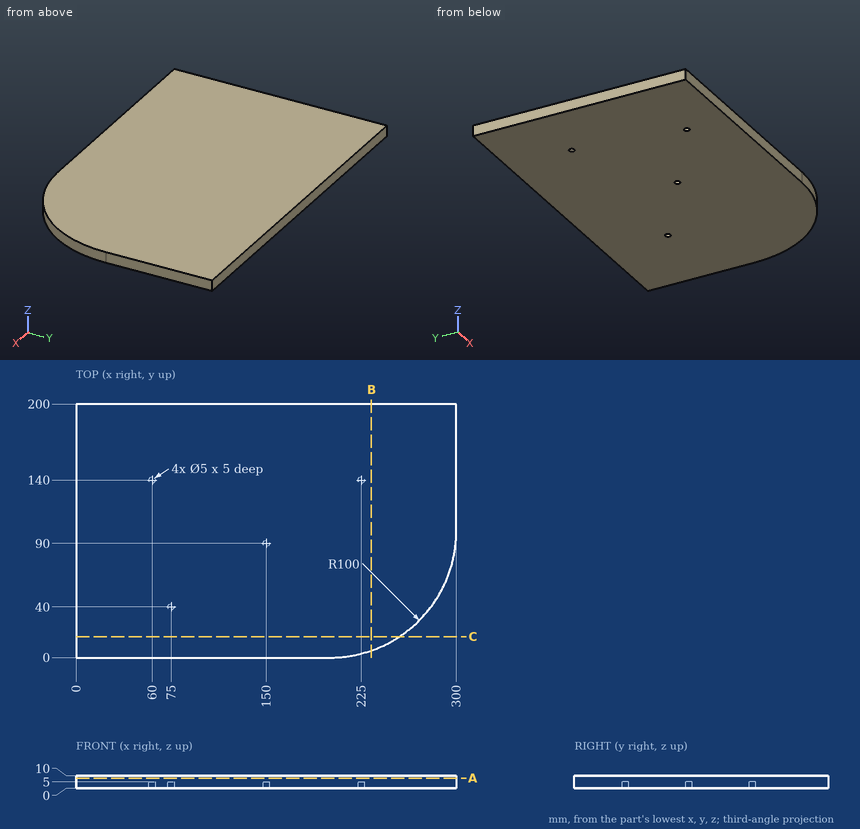
Can you work these out from the drawing? Everything is in mm from the part's minimum corner. Round coordinates to 2 decimals unless told otherwise and drop trailing zeros. Loops run counter-clockwise (first coordinate to the right, second up) from the corner with the lowest first, then second, coordinate; pieces in that order, holes last. Notation, with made-up numbers: (44.5, -15) - (89.5, -15) arc R35 ccw to (89.5, 18) - close; hole circle Ø6 at (-6.5, 10.25). An arc over 180 degrees is marked (long way). Answer in a Markdown table with one row per item. Add a question column.
Q1. For pin 1 Ø5.5 at (x, y) = (75, 40) entering from -Z; pin 2 Ø2.5 at (x, y) = (59.5, 139) entering from -Z; pin 3 Ø1 at (y, z) = (24, 8.5) entering from +X; pin 4 Ø2 at (y, z) = (30, 4.5) entering from +X, each with a flat end and sliding along its axis, tell me the tip position at first contact or that it passes through.
Q2. I need wall thicknesses on L1, parallel to X at y = 140, z = 1.75; L2, parallel to Y at x = 60, z = 2.3; L3, parallel to Y at x = 75, z = 1.45. Which ranges of each line are inside material? Lowest first, please.
Q3. I want a section at B-B on x = 233. List the corners of the cut face in (y, z) for me.
Q4. I want a section at C-C on y = 16.5. List the corners of the cut face in (x, z) for me (3 decimals), and give its area (3 significant figures).
Q5. I want a section at A-A on z = 8. List the corners of the cut face in (x, y) for me.
A:
| question | item | result |
|---|---|---|
| 1 | pin 1 | z = 0 |
| 1 | pin 2 | z = 5 |
| 1 | pin 3 | x = 265.57 |
| 1 | pin 4 | x = 272.38 |
| 2 | L1 | 0 to 57.5, 62.5 to 222.5, 227.5 to 300 |
| 2 | L2 | 0 to 137.5, 142.5 to 200 |
| 2 | L3 | 0 to 37.5, 42.5 to 200 |
| 3 | outline | (5.6, 0) - (200, 0) - (200, 10) - (5.6, 10) - close |
| 4 | outline | (0, 0) - (255.025, 0) - (255.025, 10) - (0, 10) - close |
| 4 | area | 2,550 mm^2 |
| 5 | outline | (0, 0) - (200, 0) arc R100 ccw to (300, 100) - (300, 200) - (0, 200) - close |
